from build123d import *

# Parameters (mm, degrees)
SKETCH2_R           = 2
SKETCH2_R_2         = 1.999999991
BOSS_EXTRUDE1_DEPTH = 5.588
SKETCH7_R           = 2.032
CUT_EXTRUDE1_DEPTH  = 5.588


with BuildPart() as part:
    # Sketch2 → Boss-Extrude1 (new body)
    with BuildSketch(Plane(origin=(0, 0, 0), x_dir=(1, 0, 0), z_dir=(0, 1, 0))):
        with BuildLine():
            ThreePointArc((17.295902343, -30.526810701), (16.688093876, -28.878103365), (15.15555913, -28.018449791))
            Line((15.15555913, -28.018449791), (13.238676936, -27.713033224))
            ThreePointArc((13.238676936, -27.713033224), (11.241051513, -26.538356195), (10.573787778, -24.319092227))
            Line((10.573787778, -24.319092227), (12.5603, 0))
            ThreePointArc((12.5603, 0), (0.603657177, 12.545785512), (-12.502275592, 1.2059192))
            Line((-12.502275592, 1.2059192), (-16.498266045, -40.222207921))
            ThreePointArc((-16.498266045, -40.222207921), (-16.507064815, -40.344000039), (-16.51, -40.466074291))
            Line((-16.51, -40.466074291), (-16.51, -221.328861788))
            ThreePointArc((-16.51, -221.328861788), (-12.970187584, -225.680718913), (-7.988667969, -223.101301399))
            Line((-7.988667969, -223.101301399), (16.979901226, -165.677523619))
            ThreePointArc((16.979901226, -165.677523619), (17.216065593, -164.934164738), (17.295902343, -164.158289667))
            Line((17.295902343, -164.158289667), (17.295902343, -30.526810701))
        make_face()
        with Locations(Location((-11.43, -219.075, 0), (0, 0, 270))):
            Circle(SKETCH2_R, mode=Mode.SUBTRACT)
        with Locations(Location((-11.43, -212.725, 0), (0, 0, 270))):
            Circle(SKETCH2_R, mode=Mode.SUBTRACT)
        with Locations(Location((-11.43, -206.375, 0), (0, 0, 270))):
            Circle(SKETCH2_R, mode=Mode.SUBTRACT)
        with Locations(Location((-11.43, -200.025, 0), (0, 0, 270))):
            Circle(SKETCH2_R, mode=Mode.SUBTRACT)
        with BuildLine():
            ThreePointArc((7.135902343, -162.410770806), (8.023611961, -165.648962244), (10.438542905, -167.981776143))
            Line((10.438542905, -167.981776143), (-0.534170778, -193.217289931))
            ThreePointArc((-0.534170778, -193.217289931), (-2.234040931, -194.665234867), (-4.420389569, -194.211381682))
            Line((-4.420389569, -194.211381682), (-11.716886202, -188.551043102))
            ThreePointArc((-11.716886202, -188.551043102), (-12.441018517, -187.661516081), (-12.7, -186.544128716))
            Line((-12.7, -186.544128716), (-12.7, -149.615408258))
            ThreePointArc((-12.7, -149.615408258), (-11.988693683, -148.474898999), (-10.651556899, -148.611951065))
            Line((-10.651556899, -148.611951065), (7.135902343, -162.410770806))
        make_face(mode=Mode.SUBTRACT)
        with BuildLine():
            ThreePointArc((10.656105825, -153.315833936), (9.771695946, -153.639779081), (8.923603828, -154.049487576))
            Line((8.923603828, -154.049487576), (-10.733772403, -138.80005889))
            ThreePointArc((-10.733772403, -138.80005889), (-12.182037035, -137.021004847), (-12.7, -134.786230117))
            Line((-12.7, -134.786230117), (-12.7, -90.4875))
            ThreePointArc((-12.7, -90.4875), (-11.803536501, -90.43671411), (-10.918544548, -90.285006317))
            Line((-10.918544548, -90.285006317), (10.027134635, -128.362607876))
            ThreePointArc((10.027134635, -128.362607876), (10.49635106, -129.547067395), (10.656105825, -130.811024207))
            Line((10.656105825, -130.811024207), (10.656105825, -153.315833936))
        make_face(mode=Mode.SUBTRACT)
        with Locations(Location((13.485902343, -162.410770806, 0), (0, 0, 270))):
            Circle(SKETCH2_R, mode=Mode.SUBTRACT)
        with BuildLine():
            Line((-10.16, -44.337182032), (1.663048834, -44.337182032))
            ThreePointArc((1.663048834, -44.337182032), (2.739129831, -44.932682449), (2.806066447, -46.160725831))
            Line((2.806066447, -46.160725831), (-11.055993219, -74.784618621))
            ThreePointArc((-11.055993219, -74.784618621), (-11.873503915, -74.655646925), (-12.7, -74.6125))
            Line((-12.7, -74.6125), (-12.7, -46.877182032))
            ThreePointArc((-12.7, -46.877182032), (-11.956051224, -45.081130808), (-10.16, -44.337182032))
        make_face(mode=Mode.SUBTRACT)
        with BuildLine():
            ThreePointArc((-9.903213406, -40.527182032), (-11.783508673, -39.694838236), (-12.431479451, -37.743315662))
            Line((-12.431479451, -37.743315662), (-9.755434212, -9.99962016))
            ThreePointArc((-9.755434212, -9.99962016), (-2.756273581, -13.695395429), (5.127655889, -12.99492382))
            Line((5.127655889, -12.99492382), (3.069264048, -38.19397392))
            ThreePointArc((3.069264048, -38.19397392), (2.259083254, -39.854914801), (0.537695935, -40.527182032))
            Line((0.537695935, -40.527182032), (-9.903213406, -40.527182032))
        make_face(mode=Mode.SUBTRACT)
        with BuildLine():
            ThreePointArc((2.999946232, -3.71521973), (-4.455639512, 1.717501551), (4.717447783, 0.740419782))
            Line((4.717447783, 0.740419782), (2.999946232, -3.71521973))
        make_face(mode=Mode.SUBTRACT)
        with BuildLine():
            ThreePointArc((-8.804706991, -86.222769023), (-8.262040897, -82.55), (-8.804706991, -78.877230977))
            Line((-8.804706991, -78.877230977), (7.575478058, -45.053638233))
            ThreePointArc((7.575478058, -45.053638233), (8.043996088, -44.531101035), (8.718495671, -44.337182032))
            Line((8.718495671, -44.337182032), (10.945902343, -44.337182032))
            ThreePointArc((10.945902343, -44.337182032), (11.843927955, -44.70915642), (12.215902343, -45.607182032))
            Line((12.215902343, -45.607182032), (12.215902343, -62.618124667))
            ThreePointArc((12.215902343, -62.618124667), (6.881902343, -71.709053992), (12.215902343, -80.799983318))
            Line((12.215902343, -80.799983318), (12.215902343, -119.492817968))
            ThreePointArc((12.215902343, -119.492817968), (11.261891546, -120.722879277), (9.83314514, -120.104922051))
            Line((9.83314514, -120.104922051), (-8.804706991, -86.222769023))
        make_face(mode=Mode.SUBTRACT)
        with Locations(Location((13.485902343, -38.1, 0), (0, 0, 270))):
            Circle(SKETCH2_R_2, mode=Mode.SUBTRACT)
    extrude(amount=BOSS_EXTRUDE1_DEPTH)

    # Sketch7 → Cut-Extrude1 (cut)
    with BuildSketch(Plane(origin=(0, 5.588, 0), x_dir=(1, 0, 0), z_dir=(0, 1, 0))):
        with Locations(Location((12.215902343, -71.655983318, 0), (0, 0, 270))):
            Circle(SKETCH7_R)
    extrude(amount=-CUT_EXTRUDE1_DEPTH, mode=Mode.SUBTRACT)


solid = part.part
Can you work these out from the model? Positions are in its coordinate system, mm. Coordinates: 2 decimals unless noted, no trailing zeros. Loops run counter-clockwise (first coordinate to the right, second up) from the corner with the lowest first, then second, coordinate; pieces in that order, holes last. Notation, with made-up numbers: (87, 36) - (125, 36) arc R22 ccw to (125, 71) - close; hole circle Ø4 at (6, -36.75). An arc over 180 degrees is marked (long way). Answer as a JSON object with one key per item and string values. Group by question number.
Item 1: If we section it at B-B (y = 3.95): State how many separate pieces and enclosed holes the cut face has, plus the area to 3 significant figures.
Item 2: If we mould it in two halves opening along Z, with no side actions, what happens to faces 1 (the face through (-14.472, 2.755, 19.218)), 2 (the face through (4.32, 2.75, 194.79)), 3 (the face through (12.216, 3, 54))? For each: released by +Z, released by -Z, zero draft, split by the parting line, or undercut.
Item 3: If we section it at A-A (z = 66): List the corners of the cut face in (x, y) for me, plus the area to 3 significant figures.
Item 4: For pin 1 (2.5 mm diameter, centred on x = 10, y = 3.5, fed in from +Z) (3 decimals), with a flat end and sliding along its axis, tell me the tip position at first contact or that it passes through.
Item 5: If I drill on L1, parallel to X at y = 4, z = 60.5; L2, parallel to Z at x = 8, y = 3.2; L3, parallel to X at y = 2.15, z = 49.5, over which ranges is the centre line in solid material (lowest first)? Write a range as from..to.
Returned:
{
 "1": {"separate pieces": "1", "enclosed holes": "13", "area": "3,480 mm²"},
 "2": {"face 1": "released by -Z", "face 2": "released by +Z", "face 3": "undercut"},
 "3": {"outline": "(-16.51, 0) - (-12.7, 0) - (-12.7, 5.59) - (-16.51, 5.59) - close; (-6.8, 0) - (-2.57, 0) - (-2.57, 5.59) - (-6.8, 5.59) - close; (8.59, 0) - (17.3, 0) - (17.3, 5.59) - (8.59, 5.59) - close", "area": "93.6 mm²"},
 "4": {"pin 1": "stops at z = 184.605"},
 "5": {"L1": "x = -16.51..-12.7, -4.14..0.1, 12.22..17.3", "L2": "z = -9.68..44.56, 67.01..76.4, 116.77..124.68, 153.33..165.61, 173.59..186.33", "L3": "x = -16.51..-12.7, 1.19..5.42, 12.22..17.3"}
}
